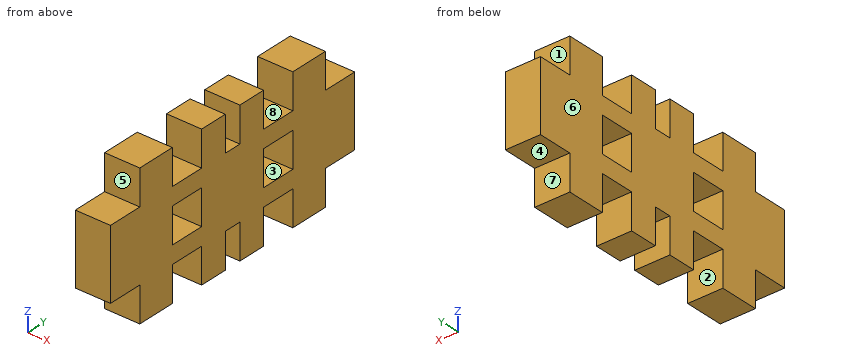
```python
from build123d import *

# Parameters (mm, degrees)
SKETCH1_R                = 8
SKETCH1_R_2              = 4
BOSS_EXTRUDE1_DEPTH      = 9
BOSS_EXTRUDE1_2_DEPTH    = 9
SKETCH2_R                = 4
BOSS_EXTRUDE3_DEPTH      = 9
FILLET1_R                = 1
CUT_EXTRUDE1_DEPTH       = 214.789616212
SKETCH4_W                = 9
SKETCH4_H                = 27
BOSS_EXTRUDE4_DEPTH      = 75
BOSS_EXTRUDE5_START      = 9
SKETCH5_R                = 25
SKETCH5_R_2              = 4
BOSS_EXTRUDE5_DEPTH      = 9
BOSS_EXTRUDE6_DEPTH      = 4.5
BOSS_EXTRUDE6_DEPTH_BACK = 4.5
BOSS_EXTRUDE7_DEPTH      = 4.5
BOSS_EXTRUDE7_DEPTH_BACK = 4.5
BOSS_EXTRUDE7_START      = -25
SKETCH9_W                = 9
SKETCH9_H                = 7
SKETCH9_H_2              = 9
CUT_EXTRUDE2_DEPTH       = 217.612557346
CUT_EXTRUDE3_DEPTH       = 216.299790989
CUT_EXTRUDE3_DEPTH_BACK  = 216.299790989
SKETCH10_W               = 383.266903908
SKETCH10_H               = 66.559710411
SKETCH10_W_2             = 9
SKETCH10_H_2             = 36
SKETCH12_W               = 9
SKETCH12_H               = 9
SKETCH12_W_2             = 4.5
SKETCH12_H_2             = 9.054007778
SKETCH12_H_3             = 4.5
SKETCH12_H_4             = 5
CUT_EXTRUDE4_DEPTH       = 81.218451743


with BuildPart() as part:
    # Sketch1 → Boss-Extrude1 (new body)
    with BuildSketch(Plane.XY):
        with Locations((-125, 0)):
            Circle(SKETCH1_R)
        with Locations((-125, 0)):
            Circle(SKETCH1_R_2, mode=Mode.SUBTRACT)
    extrude(amount=BOSS_EXTRUDE1_DEPTH)



with BuildPart() as body_2:
    # Sketch1 → Boss-Extrude1 2 (new body)
    with BuildSketch(Plane.XY):
        with Locations((125, 0)):
            Circle(SKETCH1_R)
        with Locations((125, 0)):
            Circle(SKETCH1_R_2, mode=Mode.SUBTRACT)
    extrude(amount=BOSS_EXTRUDE1_2_DEPTH)


with BuildPart() as part_1:
    add(part.part)

    add(body_2.part)  # Boss-Extrude3 merges body 2
    # Sketch2 → Boss-Extrude3 (add)
    with BuildSketch(Plane.XY):
        with BuildLine():
            Line((-175, -75), (125, -75))
            ThreePointArc((125, -75), (130.131670325, -43.377223009), (145.000000492, -14.999999344))
            ThreePointArc((145.000000492, -14.999999344), (143.981414944, 16.269784471), (113.235294528, 22.058823748))
            ThreePointArc((113.235294528, 22.058823748), (25.000000075, 0), (-63.235294395, 22.058823677))
            ThreePointArc((-63.235294395, 22.058823677), (-75.420498385, 24.996463372), (-87.499999896, 21.650635154))
            ThreePointArc((-87.499999896, 21.650635154), (-99.999999954, 18.301270189), (-112.500000024, 21.650635108))
            ThreePointArc((-112.500000024, 21.650635108), (-124.99999995, 25), (-137.49999989, 21.650635158))
            ThreePointArc((-137.49999989, 21.650635158), (-149.999999954, 18.301270189), (-162.50000003, 21.650635112))
            ThreePointArc((-162.50000003, 21.650635112), (-193.705072901, 16.586749162), (-195.000000551, -14.999999265))
            ThreePointArc((-195.000000551, -14.999999265), (-180.13167034, -43.377222962), (-175, -75))
        make_face()
        with Locations((125, 0)):
            Circle(SKETCH2_R, mode=Mode.SUBTRACT)
        with Locations((-175, 0)):
            Circle(SKETCH2_R, mode=Mode.SUBTRACT)
        with Locations((-125, 0)):
            Circle(SKETCH2_R, mode=Mode.SUBTRACT)
        with Locations((-75, 0)):
            Circle(SKETCH2_R, mode=Mode.SUBTRACT)
    extrude(amount=BOSS_EXTRUDE3_DEPTH)

    # Fillet1
    fillet1_edges = [part_1.edges().sort_by_distance(p)[0] for p in [
        (-175, -75, 4.5),
        (125, -75, 4.5),
    ]]
    fillet(fillet1_edges, radius=FILLET1_R)

    # Sketch3 → Cut-Extrude1 (cut, through all)
    with BuildSketch(Plane.XY):
        Polygon((25, 0), (25, -75), (150, -75), (150, 25), (25, 25), align=None)
    extrude(amount=CUT_EXTRUDE1_DEPTH, mode=Mode.SUBTRACT)

    # Sketch4 → Boss-Extrude4 (add)
    with BuildSketch(Plane.XZ.offset(75)):
        with Locations((25, -4.5)):
            Rectangle(SKETCH4_W, SKETCH4_H)
    extrude(amount=-BOSS_EXTRUDE4_DEPTH)

    # Sketch5 → Boss-Extrude5 (add)
    # profile 1 of 4: a face of its own
    with BuildSketch(Plane(origin=(0, 0, -18), x_dir=(-1, 0, 0), z_dir=(0, 0, -1)).offset(BOSS_EXTRUDE5_START)):
        with BuildLine():
            ThreePointArc((-145.000000304, -14.999999594), (-130.131670275, -43.377223158), (-125, -75))
            Line((-125, -75), (-29.5, -75))
            Line((-29.5, -75), (-29.5, 0))
            Line((-29.5, 0), (-100, 0))
            ThreePointArc((-100, 0), (-117.09430609, -23.717082532), (-145.000000304, -14.999999594))
        make_face()
    # profile 2 of 4: a face of its own
    with BuildSketch(Plane(origin=(0, 0, -18), x_dir=(-1, 0, 0), z_dir=(0, 0, -1)).offset(BOSS_EXTRUDE5_START)):
        with Locations((-125, 0)):
            Circle(SKETCH5_R)
        with Locations((-125, 0)):
            Circle(SKETCH5_R_2, mode=Mode.SUBTRACT)
    # profile 3 of 4: a face of its own
    with BuildSketch(Plane(origin=(0, 0, -18), x_dir=(-1, 0, 0), z_dir=(0, 0, -1)).offset(BOSS_EXTRUDE5_START)):
        Polygon((-29.5, 0), (-29.5, -75), (-20.5, -75), (-20.5, 0), (-25, 0), align=None)
    # profile 4 of 4: a face of its own
    with BuildSketch(Plane(origin=(0, 0, -18), x_dir=(-1, 0, 0), z_dir=(0, 0, -1)).offset(BOSS_EXTRUDE5_START)):
        with BuildLine():
            Line((-100, 0), (-29.5, 0))
            Line((-29.5, 0), (-25, 0))
            ThreePointArc((-25, 0), (-70.475429529, 5.598281181), (-113.235293817, 22.058823369))
            ThreePointArc((-113.235293817, 22.058823369), (-103.56267677, 12.86239374), (-100, 0))
        make_face()
    extrude(amount=-BOSS_EXTRUDE5_DEPTH)

    # Sketch7 → Boss-Extrude6 (add, two sides: drawn at the far end of the back side and taken through both)
    with BuildSketch(Plane(origin=(0, -25, 0), x_dir=(1, 0, 0), z_dir=(0, 1, 0)).offset(-BOSS_EXTRUDE6_DEPTH_BACK)):
        with BuildLine():
            Line((56.5, 18), (29.5, 18))
            Line((29.5, 18), (29.5, -9))
            ThreePointArc((29.5, -9), (48.591883092, -1.091883092), (56.5, 18))
        make_face()
        with BuildLine():
            Line((-6.5, 0), (20.5, 0))
            Line((20.5, 0), (20.5, 27))
            ThreePointArc((20.5, 27), (1.408116908, 19.091883092), (-6.5, 0))
        make_face()
    extrude(amount=BOSS_EXTRUDE6_DEPTH + BOSS_EXTRUDE6_DEPTH_BACK)

    # Sketch7<3> → Boss-Extrude7 (add, two sides: drawn at the far end of the back side and taken through both)
    with BuildSketch(Plane(origin=(0, -25, 0), x_dir=(1, 0, 0), z_dir=(0, 1, 0)).offset(BOSS_EXTRUDE7_START - BOSS_EXTRUDE7_DEPTH_BACK)):
        with BuildLine():
            Line((56.5, 18), (29.5, 18))
            Line((29.5, 18), (29.5, -9))
            ThreePointArc((29.5, -9), (48.591883092, -1.091883092), (56.5, 18))
        make_face()
        with BuildLine():
            Line((-6.5, 0), (20.5, 0))
            Line((20.5, 0), (20.5, 27))
            ThreePointArc((20.5, 27), (1.408116908, 19.091883092), (-6.5, 0))
        make_face()
    extrude(amount=BOSS_EXTRUDE7_DEPTH + BOSS_EXTRUDE7_DEPTH_BACK)

    # Sketch9 → Cut-Extrude2 (cut, through all)
    with BuildSketch(Plane.XY.offset(9)):
        with Locations((-160.208548161, -53.5)):
            Rectangle(SKETCH9_W, SKETCH9_H)
        with Locations((-160.208548161, -70.5)):
            Rectangle(SKETCH9_W, SKETCH9_H_2)
        with Locations((-25.351798772, -53.5)):
            Rectangle(SKETCH9_W, SKETCH9_H)
        with Locations((-25.351798772, -70.5)):
            Rectangle(SKETCH9_W, SKETCH9_H_2)
        with Locations((109.504950616, -53.5)):
            Rectangle(SKETCH9_W, SKETCH9_H)
        with Locations((109.504950616, -70.5)):
            Rectangle(SKETCH9_W, SKETCH9_H_2)
    extrude(amount=-CUT_EXTRUDE2_DEPTH, mode=Mode.SUBTRACT)

    # Sketch10 → Cut-Extrude3 (cut, two sides: drawn at the far end of the back side and taken through both)
    with BuildSketch(Plane(origin=(0, 0, 0), x_dir=(1, 0, 0), z_dir=(0, 1, 0)).offset(-CUT_EXTRUDE3_DEPTH_BACK)):
        with Locations((-25.802694846, 3.514309581)):
            Rectangle(SKETCH10_W, SKETCH10_H)
        with Locations((25, 9)):
            Rectangle(SKETCH10_W_2, SKETCH10_H_2, mode=Mode.SUBTRACT)
    extrude(amount=CUT_EXTRUDE3_DEPTH + CUT_EXTRUDE3_DEPTH_BACK, mode=Mode.SUBTRACT)

    # Sketch12 → Cut-Extrude4 (cut, through all)
    with BuildSketch(Plane.ZY.offset(-20.5)):
        with Locations((-22.5, -23.5)):
            Rectangle(SKETCH12_W, SKETCH12_H)
        with Locations((-22.5, -51.5)):
            Rectangle(SKETCH12_W, SKETCH12_H)
        with Locations((4.5, -51.5)):
            Rectangle(SKETCH12_W, SKETCH12_H)
        with Locations((4.5, -23.5)):
            Rectangle(SKETCH12_W, SKETCH12_H)
        with Locations((-6.75, -23.5)):
            Rectangle(SKETCH12_W_2, SKETCH12_H)
        with Locations((-11.25, -23.5)):
            Rectangle(SKETCH12_W_2, SKETCH12_H)
        with Locations((-11.25, -51.5)):
            Rectangle(SKETCH12_W_2, SKETCH12_H)
        with Locations((-6.75, -51.5)):
            Rectangle(SKETCH12_W_2, SKETCH12_H)
        with Locations((-22.5, -4.5)):
            Rectangle(SKETCH12_W, SKETCH12_H)
        with Locations((4.5, -4.472996111)):
            Rectangle(SKETCH12_W, SKETCH12_H_2)
        with Locations((4.5, -70.5)):
            Rectangle(SKETCH12_W, SKETCH12_H)
        with Locations((-22.5, -70.5)):
            Rectangle(SKETCH12_W, SKETCH12_H)
        with Locations((-22.5, -37.5)):
            Rectangle(SKETCH12_W, SKETCH12_H_3)
        with Locations((4.5, -37.5)):
            Rectangle(SKETCH12_W, SKETCH12_H_3)
        with Locations((-22.5, 2.5)):
            Rectangle(SKETCH12_W, SKETCH12_H_4)
    extrude(amount=-CUT_EXTRUDE4_DEPTH, mode=Mode.SUBTRACT)


solid = part_1.part
```
Work out the finished part from the listing and answer in its coordinate system (mm). Face numbers are marked on the shaded views. A direction names the side the tool comes from. Coordinates: 2 decimals unless noted, no trailing zeros. Order: outer loops, then holes, each group sorted by start corner. A loop starts at its lowest first (then second) coordinate and runs counter-clockwise, first axis right, second up. Notation, with made-up numbers: M 47.25,31 L 68.25,31 A33 cw 68.25,68 Z; hole C 31,9 d3. An arc over 180 degrees is marked long. Use CSV: the item, a comma, the result in double quotes.
1) Section D-D on x = 24 is taken. Count the separate pieces of the cut face and the enclosed holes in it, plus the area to 3 significant figures.
Worked out:
separate pieces,"1"
enclosed holes,"2"
area,"1,810 mm^2"
2) Section B-B on y = -52 is taken. Write down the section's boundary in (x, z), plus the area to 3 significant figures.
Worked out:
outline,"M 20.5,-18 L 29.5,-18 L 29.5,-13.5 L 20.5,-13.5 Z; M 20.5,-4.5 L 29.5,-4.5 L 29.5,0 L 20.5,0 Z"
area,"81.0 mm^2"
3) Consider line 1 (Y direction, x = 24.75, z = -7.5); line 2 (Y direction, x = 27.25, z = 1); line 3 (Z direction, x = 27.5, y = -48). Determine where each line is inside the solid, lowest interval first. Write a range as [from, to].
Worked out:
line 1,"y = [-75, -56], [-47, -28], [-19, 0]"
line 2,"y = [-66, -56], [-47, -39.75], [-35.25, -28], [-19, -9]"
line 3,"z = [-18, -13.5], [-4.5, 0]"
4) For the marked faces 1, 2, 3 and 4, determine the directions among +Z, -Z, +X, -X, +Y, -Y from which every point of the face is accessible in a straight line to the end or side of a thin tool.
Worked out:
face 1,"+Z, +X, -X, +Y"
face 2,"-Z, +X, -X"
face 3,"+X, -X"
face 4,"-Z, +X, -X, +Y"
5) Section C-C on z = -11.5 is taken. Write down the section's boundary in (x, y), plus the area to 3 significant figures.
Worked out:
outline,"M 20.5,-75 L 29.5,-75 L 29.5,-56 L 20.5,-56 Z; M 20.5,-47 L 29.5,-47 L 29.5,-28 L 20.5,-28 Z; M 20.5,-19 L 29.5,-19 L 29.5,0 L 20.5,0 Z"
area,"513 mm^2"
6) Section A-A on z = 4.5 is taken. Write down the section's boundary in (x, y).
Worked out:
outline,"M 20.5,-66 L 29.5,-66 L 29.5,-56 L 20.5,-56 Z; M 20.5,-47 L 29.5,-47 L 29.5,-39.75 L 20.5,-39.75 Z; M 20.5,-35.25 L 29.5,-35.25 L 29.5,-28 L 20.5,-28 Z; M 20.5,-19 L 29.5,-19 L 29.5,-9 L 20.5,-9 Z"
7) Flat-ended cylindrical pins translate along their axes: pin 1 Ø3 at (x, z) = (24.5, -11.5) entering from +Y; pin 2 Ø2.5 at (x, z) = (23, -23) entering from -Y; pin 3 Ø4.5 at (x, y) = (24, -50) entering from +Z; pin 4 Ø4.5 at (x, y) = (26.5, -25) entering from -Z. Find the tip coordinate at first contact, or state that the pin passes through.
Worked out:
pin 1,"stops at y = 0"
pin 2,"stops at y = -66"
pin 3,"stops at z = 0"
pin 4,"stops at z = -18"
8) Determine the mould class of the marked faces 5, 6, 7 and 8 for opening direction Y: released by +Y, released by -Y, zero draft, split by the parting line, or undercut.
Worked out:
face 5,"released by -Y"
face 6,"zero draft"
face 7,"released by +Y"
face 8,"undercut"
